from build123d import *

# Parameters (mm, degrees)
EXTRUDE_2_DEPTH          = 38
SKETCH_2_R               = 11
EXTRUDE_3_DEPTH          = 2
FILLET_1_R               = 1
SKETCH_3_R               = 2.5
EXTRUDE_4_DEPTH          = 24
SKETCH_4_R               = 1.5
CUT_EXTRUDE_1_DEPTH      = 4.5
PATTERN_CIRCULAR_1_COUNT = 4


with BuildPart() as part:
    # 草图1 → 凸台-拉伸2 (new body)
    with BuildSketch(Plane(origin=(0, 0, 0), x_dir=(0, 0, -1), z_dir=(1, 0, 0))):
        Polygon((0, 40.3), (2, 42.3), (40.3, 42.3), (42.3, 40.3), (42.3, 2), (40.3, 0), (2, 0), (0, 2), align=None)
    extrude(amount=EXTRUDE_2_DEPTH)

    # 草图2 → 凸台-拉伸3 (add)
    with BuildSketch(Plane.ZY):
        with Locations((-21.15, 21.15)):
            Circle(SKETCH_2_R)
    extrude(amount=EXTRUDE_3_DEPTH)

    # 圆角1
    fillet_1_edges = [part.edges().sort_by_distance(p)[0] for p in [
        (-2, 21.15, -32.15),
    ]]
    fillet(fillet_1_edges, radius=FILLET_1_R)

    # 草图3 → 凸台-拉伸4 (add)
    with BuildSketch(Plane.ZY.offset(2)):
        with Locations((-21.15, 21.15)):
            Circle(SKETCH_3_R)
    extrude(amount=EXTRUDE_4_DEPTH)

    # 草图4 → 切除-拉伸1 (cut)
    with BuildSketch(Plane.ZY):
        with Locations((-36.65, 36.65)):
            Circle(SKETCH_4_R)
    cut_extrude_1 = extrude(amount=-CUT_EXTRUDE_1_DEPTH, mode=Mode.SUBTRACT)

    # 阵列(圆周)1: 切除-拉伸1 ×4 about axis
    pattern_circular_1_axis = Axis((0, 21.15, -21.15), (1, 0, 0))
    for i in range(1, PATTERN_CIRCULAR_1_COUNT):
        add(cut_extrude_1.rotate(pattern_circular_1_axis, i * 360 / PATTERN_CIRCULAR_1_COUNT), mode=Mode.SUBTRACT)


solid = part.part
Could you check a few things on this model? Use its own coordinates, in mm. A direction names the side the tool comes from. Give positions to 0.01 mm unless a question says otherwise; leave off trailing zeros. Loops run counter-clockwise (first coordinate to the right, second up) from the corner with the lowest first, then second, coordinate; pieces in that order, holes last. Notation, with made-up numbers: (11.5, 1.5) -> (38.5, 1.5) arc R15 cw to (38.5, 10.5) -> close; hole circle Ø10 at (85.5, 49). An arc over 180 degrees is marked (long way). Return JSON: item names as keys, results as strings.
Item 1: If we section it at B-B on z = -5.65: List the corners of the cut face in (x, y) for me, plus the area to 3 significant figures.
Geometry results:
{"outline": "(0, 0) -> (38, 0) -> (38, 42.3) -> (0, 42.3) -> (0, 38.15) -> (4.5, 38.15) -> (4.5, 35.15) -> (0, 35.15) -> (0, 7.15) -> (4.5, 7.15) -> (4.5, 4.15) -> (0, 4.15) -> close", "area": "1,580 mm²"}
Item 2: If we section it at A-A on y = 21.15: List the corners of the cut face in (x, z) for me, plus the area to 3 significant figures.
Geometry results:
{"outline": "(-26, -23.65) -> (-2, -23.65) -> (-2, -31.15) arc R1 ccw to (-1, -32.15) -> (0, -32.15) -> (0, -42.3) -> (38, -42.3) -> (38, 0) -> (0, 0) -> (0, -10.15) -> (-1, -10.15) arc R1 ccw to (-2, -11.15) -> (-2, -18.65) -> (-26, -18.65) -> close", "area": "1,770 mm²"}
Item 3: If we section it at D-D on x = -4: List the corners of the cut face in (y, z) for me, plus the area to 3 significant figures.
Geometry results:
{"outline": "circle Ø5 at (21.15, -21.15)", "area": "19.6 mm²"}
Item 4: Which directions (+Z, -Z, +X, -X, +Y, -Y) give clear straight access to the entire face, cutting with the end or side of a thin tool? Please do faces 4 (the flat face through (18.7, 1, -41.3)), 5 (the flat face through (4.5, 6, -6)).
Geometry results:
{"face 4": "-Z, +X, -X, -Y", "face 5": "-X"}
Item 5: If we section it at C-C on y = 5.65: List the corners of the cut face in (x, z) for me, plus the area to 3 significant figures.
Geometry results:
{"outline": "(0, -42.3) -> (38, -42.3) -> (38, 0) -> (0, 0) -> (0, -4.15) -> (4.5, -4.15) -> (4.5, -7.15) -> (0, -7.15) -> (0, -35.15) -> (4.5, -35.15) -> (4.5, -38.15) -> (0, -38.15) -> close", "area": "1,580 mm²"}
Item 6: I need wall thicknesses on L1, parallel to Y at x = 2, z = -36; L2, parallel to Z at x = 2, y = 36; L3, parallel to X at y = 36.5, z = -26. Which ranges of each line are inside material? Lowest first, please. Write a range as from..to.
Geometry results:
{"L1": "y = 0..4.3, 7..35.3, 38..42.3", "L2": "z = -42.3..-38, -35.3..-7, -4.3..0", "L3": "x = 0..38"}
Item 7: I'm going to push flat-ended pins straight in: pin 1 (10 mm diameter, centred on x = -9.5, y = 10, fed in from -Z); pin 2 (2.5 mm diameter, centred on y = 36.5, z = -37.5, fed in from -X); pin 3 (1.5 mm diameter, centred on y = 17, z = -19, fed in from -X); pin 4 (1.5 mm diameter, centred on y = 37, z = -6, fed in from -X). Where does each tip first touch, or does it pass through?
Geometry results:
{"pin 1": "passes through", "pin 2": "stops at x = 0", "pin 3": "stops at x = -2", "pin 4": "stops at x = 4.5"}
Item 8: We'd pull the mould along Z, two halves only. Please class faces 1 (the flat face through (4.5, 37, -6)), 2 (the flat face through (-26, 21, -21)), 3 (the flat face through (18.7, 41.3, -1)): +Z half, -Z half, draft (parallel to the pull), parting line (faces both ways), or undercut.
Geometry results:
{"face 1": "undercut", "face 2": "draft", "face 3": "+Z half"}
